The drawing under review shows one solid part. Ordinate dimensions are in mm from its lowest x, y, z. A direction names the side the tool comes from. Give positions to 0.01 mm unless a question says otherwise; leave off trailing zeros. Order: outer loops, then holes, each group sorted by start corner. A loop starts at its lowest first (then second) coordinate and runs counter-clockwise, first axis right, second up. Notation, with made-up numbers: (-23.5, -4) -> (3.5, -4) arc R24 ccw to (3.5, 8) -> close; hole circle Ø7 at (80.5, 18). An arc over 180 degrees is marked (long way). Return JSON: item names as keys, results as strings. Group by question number.
1) Add section A-A (y = 9). Give the boundary of the cut face in (x, z), then the cut area to 3 significant figures.
2) Insertion check: P1, Ø1.5, axis at x = 3, z = 10, coming from the +Y side. The pin has a flat end and moves straight along its axis. Give the tip position at first contact, or say it passes through.
3) For the marked faces 5 and 6, list the 3-axis set-ups (+Z, -Z, +X, -X, +Y, -Y) from which the entire face can be reached by the end or side of a thin tool; tool diameter is ignored.
4) Add section C-C (x = 12.25). Give the boundary of the cut face in (y, z), then the cut area to 3 significant figures.
5) The part is to be moulded in two halves that separate along X. For the marked faces 1, 2, 3 and 4, say which applies: released by +X, released by -X, zero draft, split by the parting line, or undercut.
6) To check wall thickness, follow line 1 along X through (y, z) = (8.75, 12.25); line 2 along Y through (x, z) = (4.5, 13.5); line 3 along Z through (x, y) = (1.75, 1.75). State the ranges of each line that lie inside material, in increasing order.
7) Add section B-B (z = 4.25). Give the boundary of the cut face in (x, y), then the cut area to 3 significant figures.
8) Add section D-D (z = 1.5). Give the boundary of the cut face in (x, y), then the cut area to 3 significant figures.
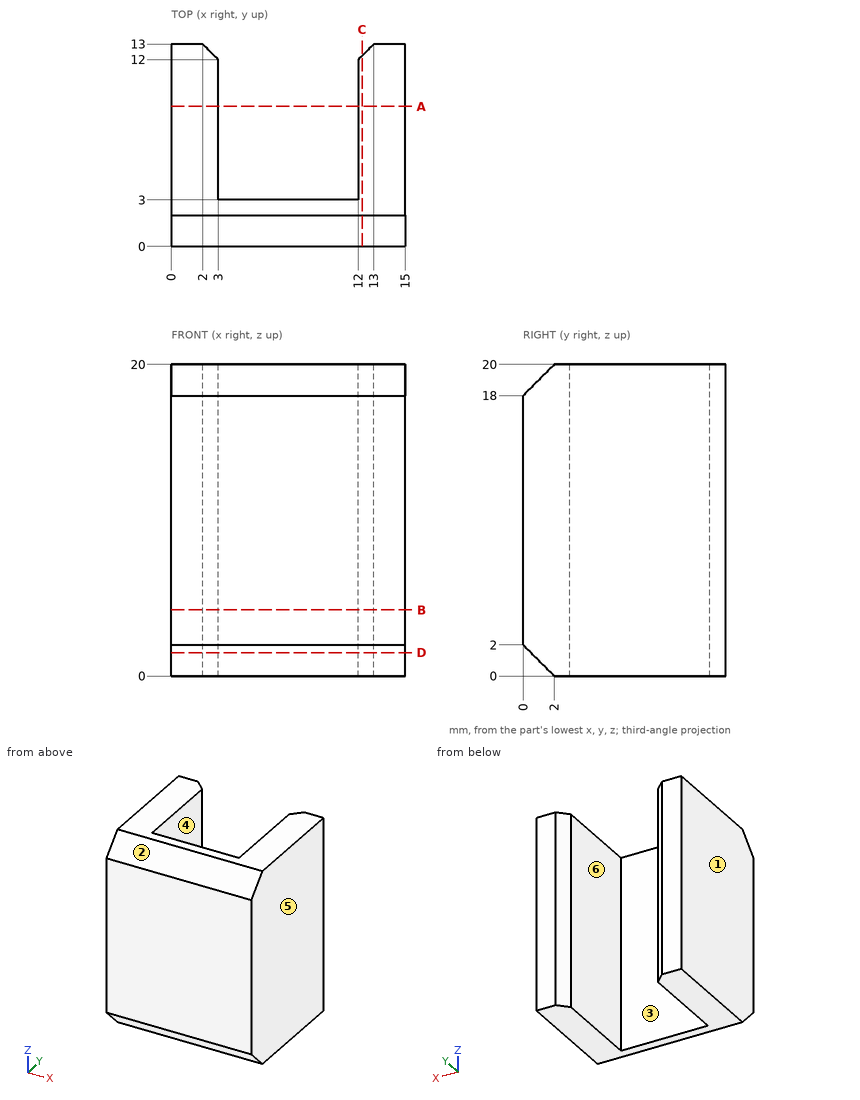
Evaluation:
{
 "1": {"outline": "(0, 0) -> (3, 0) -> (3, 20) -> (0, 20) -> close; (12, 0) -> (15, 0) -> (15, 20) -> (12, 20) -> close", "area": "120 mm^2"},
 "2": {"P1": "y = 12.75"},
 "3": {"face 5": "+Z, -Z, +X, +Y, -Y", "face 6": "+Z, -Z, +Y"},
 "4": {"outline": "(0, 2) -> (2, 0) -> (12.25, 0) -> (12.25, 20) -> (2, 20) -> (0, 18) -> close", "area": "241 mm^2"},
 "5": {"face 1": "released by -X", "face 2": "zero draft", "face 3": "undercut", "face 4": "undercut"},
 "6": {"line 1": "0 to 3, 12 to 15", "line 2": "0 to 3", "line 3": "0.25 to 19.75"},
 "7": {"outline": "(0, 0) -> (15, 0) -> (15, 13) -> (13, 13) -> (12, 12) -> (12, 3) -> (3, 3) -> (3, 12) -> (2, 13) -> (0, 13) -> close", "area": "104 mm^2"},
 "8": {"outline": "(0, 0.5) -> (15, 0.5) -> (15, 13) -> (13, 13) -> (12, 12) -> (12, 3) -> (3, 3) -> (3, 12) -> (2, 13) -> (0, 13) -> close", "area": "96.5 mm^2"}
}
